from build123d import *

# Parameters (mm, degrees)
F2_SIZE = 1


with BuildPart() as f1:
    # F0 (on Front) → F1 (revolve)
    with BuildSketch(Plane.XZ):
        Polygon((0, 30), (0, 9), (17, 9), (17, 30), (15, 30), (15, 15), (12, 15), (12, 30), (10, 30), (10, 15), (7, 15), (7, 30), (5, 30), (5, 15), (2, 15), (2, 30), align=None)
    revolve(axis=Axis((32.809981, 0, 0), (1, 0, 0)))

    # F2
    f2_edges = [f1.edges().sort_by_distance(p)[0] for p in [
        (0, 0, -9),
        (17, 0, -9),
    ]]
    chamfer(f2_edges, length=F2_SIZE)


solid = f1.part
Verification items for the finished model (mm, model axes). A direction names the side the tool comes from. Give positions to 0.01 mm unless a question says otherwise; leave off trailing zeros. Order: outer loops, then holes, each group sorted by start corner. A loop starts at its lowest first (then second) coordinate and runs counter-clockwise, first axis right, second up. Notation, with made-up numbers: (57.5, -32.75) -> (78.5, -32.75) arc R28 cw to (78.5, -11.75) -> close; hole circle Ø11 at (88.25, 89.25). An arc over 180 degrees is marked (long way). Answer as CSV lines item,"result".
Q1. Access from +Z, -Z, +X, -X, +Y, -Y to the whole of each face (thin tool, end or side, straight path). Record for faces 4 (the flat face through (2, -14, -6)), 5 (the cylindrical face through (15.99, -1.32, -29.97)).
Solutions:
face 4,"none"
face 5,"+X, -X"
Q2. Sectioned sample at B-B on x = 8.25. Record the cut outline in (y, z).
Solutions:
outline,"circle Ø30 at (0, 0); hole circle Ø18 at (0, 0)"
Q3. Sectioned sample at A-A on z = -21.5. Record the cut outline in (x, y).
Solutions:
outline,"(0, -20.92) -> (2, -20.92) -> (2, 20.92) -> (0, 20.92) -> close; (5, -20.92) -> (7, -20.92) -> (7, 20.92) -> (5, 20.92) -> close; (10, -20.92) -> (12, -20.92) -> (12, 20.92) -> (10, 20.92) -> close; (15, -20.92) -> (17, -20.92) -> (17, 20.92) -> (15, 20.92) -> close"
Q4. Depth check by flat-ended pin: pin 1 (16 mm diameter, centred on y = 0, z = 0, fed in from +X); pin 2 (4 mm diameter, centred on x = 2, z = 2, fed in from +Y); pin 3 (3 mm diameter, centred on x = 4, y = 3, fed in from +Z); pin 4 (1 mm diameter, centred on x = 10, y = 6, fed in from -Z). Enter the tip coordinate at first touch or a pass-through.
Solutions:
pin 1,"passes through"
pin 2,"stops at y = 30"
pin 3,"stops at z = 29.94"
pin 4,"stops at z = -29.49"
Q5. Release check for a two-part mould opening along Y. For faces 1 (the flat face through (7, -14, -6)), 2 (the cylindrical face through (13.479, -0.66, -14.985)), 3 (the cylindrical face through (8.605, -8.923, -1.172)) record: +Y half, -Y half, draft (parallel to the pull), parting line (faces both ways), or undercut.
Solutions:
face 1,"draft"
face 2,"parting line"
face 3,"undercut"
Q6. Scan lines: probe 1 along X at (y, z) = (24, 2.5); probe 2 along Y at (x, z) = (4.5, 0); probe 3 along Y at (x, z) = (6.25, 0). Record each from-to range of solid material in increasing order.
Solutions:
probe 1,"x = 0 to 2, 5 to 7, 10 to 12, 15 to 17"
probe 2,"y = -15 to -9, 9 to 15"
probe 3,"y = -30 to -9, 9 to 30"
